Geometry: final body of the model. Coordinates: model frame, mm. Face numbers are marked on the shaded views. A direction names the side the tool comes from. Give positions to 0.01 mm unless a question says otherwise; leave off trailing zeros. Write each loop counter-clockwise with the first axis right and the second up, starting at its lowest first coordinate (ties: lowest second). Pieces come first, ordered by that corner, then holes.
Q1. Section D-D (y = 20). Return the cut outline in (x, z).
Q2. Reachability of the marked faces 1, 2 and 3 from +Z, -Z, +X, -X, +Y, -Y: full face, straight path, thin tool, end or side. Return the list, or none.
Q3. Section A-A (x = -16.2). Return the cut outline in (y, z) (3 decimals), plus the area to 3 significant figures.
Q4. Section C-C (y = -4.75). Return the cut outline in (x, z) (3 decimals), plus the area to 3 significant figures.
Q5. Line query: line 1 (X direction, y = 17, z = 1.5); line 2 (X direction, y = -2.5, z = 7.5); line 3 (X direction, y = 18.25, z = 10.25). Output: solid intervals per line, ascending.
Q6. Pin query (flat end, axial travel): pin 1 Ø6 at (y, z) = (1.5, 8.5) entering from -X; pin 2 Ø1.5 at (x, z) = (-33, 6) entering from -Y; pin 3 Ø4 at (x, z) = (3, 5) entering from -Y. Return the tip coordinate at first contact, or that it passes through.
Q7. Section B-B (y = 16.5). Return the cut outline in (x, z).
Q8. Mould query, pull axis X, two halves, no side actions, for the marked faces 4, 5, 6 and 7. Classes: +X half, -X half, draft (parallel to the pull), parting line (faces both ways), or undercut.
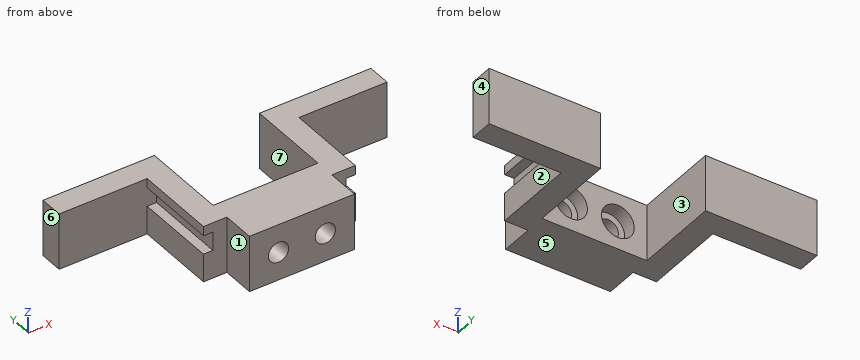
from build123d import *

# Parameters (mm, degrees)
BOSS_EXTRUDE2_DEPTH = 12
SKETCH3_W           = 4
SKETCH3_H           = 17.5
CUT_EXTRUDE1_DEPTH  = 2
SKETCH4_W           = 12
SKETCH4_H           = 11.3
BOSS_EXTRUDE3_DEPTH = 11.2
SKETCH5_R           = 3.5
CUT_EXTRUDE2_DEPTH  = 3
SKETCH6_R           = 2.165
CUT_EXTRUDE3_DEPTH  = 53.229110657


with BuildPart() as part:
    # Sketch2 → Boss-Extrude2 (new body)
    with BuildSketch(Plane.XY):
        Polygon((0, 0), (5, 0), (5, 17.5), (23.8, 17.5), (23.8, 22.5), (0, 22.5), (0, 17.5), align=None)
    boss_extrude2 = extrude(amount=BOSS_EXTRUDE2_DEPTH)

    # Sketch3 → Cut-Extrude1 (cut)
    with BuildSketch(Plane(origin=(5, 0, 0), x_dir=(0, 0, -1), z_dir=(1, 0, 0))):
        with Locations((-8, 8.75)):
            Rectangle(SKETCH3_W, SKETCH3_H)
    cut_extrude1 = extrude(amount=-CUT_EXTRUDE1_DEPTH, mode=Mode.SUBTRACT)

    # Sketch4 → Boss-Extrude3 (add)
    with BuildSketch(Plane.ZY):
        with Locations((6, -1.35)):
            Rectangle(SKETCH4_W, SKETCH4_H)
    boss_extrude3 = extrude(amount=BOSS_EXTRUDE3_DEPTH)

    # Mirror4: Boss-Extrude3 across plane
    add(boss_extrude3.mirror(Plane.ZY.offset(11.2)))

    # Mirror5: Boss-Extrude2 across plane
    add(boss_extrude2.mirror(Plane.ZY.offset(11.2)))

    # Mirror6: Cut-Extrude1 across plane
    add(cut_extrude1.mirror(Plane.ZY.offset(11.2)), mode=Mode.SUBTRACT)

    # Sketch5 → Cut-Extrude2 (cut)
    with BuildSketch(Plane(origin=(0, 4.3, 0), x_dir=(1, 0, 0), z_dir=(0, 1, 0))):
        with Locations(Location((-16.2, -6, 0), (0, 0, 270))):
            Circle(SKETCH5_R)
        with Locations(Location((-6.2, -6, 0), (0, 0, 270))):
            Circle(SKETCH5_R)
    extrude(amount=-CUT_EXTRUDE2_DEPTH, mode=Mode.SUBTRACT)

    # Sketch6 → Cut-Extrude3 (cut, through all)
    with BuildSketch(Plane(origin=(0, 1.3, 0), x_dir=(1, 0, 0), z_dir=(0, 1, 0))):
        with Locations(Location((-16.2, -6, 0), (0, 0, 270))):
            Circle(SKETCH6_R)
        with Locations(Location((-6.2, -6, 0), (0, 0, 270))):
            Circle(SKETCH6_R)
    extrude(amount=-CUT_EXTRUDE3_DEPTH, mode=Mode.SUBTRACT)


solid = part.part
Computed:
1. outline: (-46.2, 0) - (-22.4, 0) - (-22.4, 12) - (-46.2, 12) - close; (0, 0) - (23.8, 0) - (23.8, 12) - (0, 12) - close
2. face 1: +Z, -Z, -X, -Y
2. face 2: +Z, -Z, +X, -Y
2. face 3: +Z, -Z, +Y
3. outline: (-7, 0) - (4.3, 0) - (4.3, 2.5) - (1.3, 2.5) - (1.3, 3.835) - (-7, 3.835) - close; (-7, 8.165) - (1.3, 8.165) - (1.3, 9.5) - (4.3, 9.5) - (4.3, 12) - (-7, 12) - close
3. area: 78.7 mm2
4. outline: (-22.4, 0) - (0, 0) - (0, 12) - (-22.4, 12) - close; hole circle Ø4.33 at (-16.2, 6); hole circle Ø4.33 at (-6.2, 6)
4. area: 239 mm2
5. line 1: x = -27.4 to -22.4, 0 to 5
5. line 2: x = -22.4 to -17.76, -14.64 to -7.76, -4.64 to 0
5. line 3: x = -46.2 to -22.4, 0 to 23.8
6. pin 1: stops at x = -27.4
6. pin 2: stops at y = 17.5
6. pin 3: stops at y = 0
7. outline: (-27.4, 0) - (-22.4, 0) - (-22.4, 12) - (-27.4, 12) - (-27.4, 10) - (-25.4, 10) - (-25.4, 6) - (-27.4, 6) - close; (0, 0) - (5, 0) - (5, 6) - (3, 6) - (3, 10) - (5, 10) - (5, 12) - (0, 12) - close
8. face 4: +X half
8. face 5: draft
8. face 6: -X half
8. face 7: undercut
